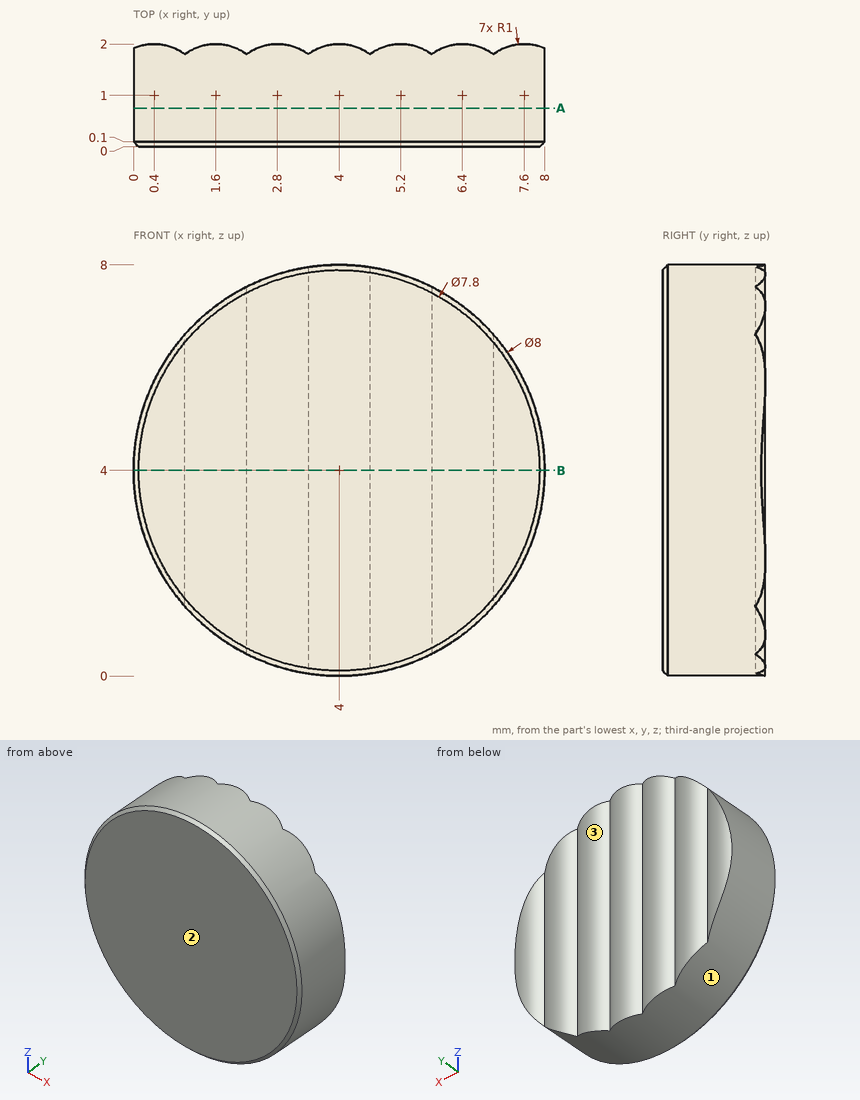
Design review of the part shown in the three views and the two pictorial views. Dimensions are in mm from the part's minimum x, y and z. Round coordinates to 2 decimals unless told otherwise and drop trailing zeros. Loops run counter-clockwise (first coordinate to the right, second up) from the corner with the lowest first, then second, coordinate; pieces in that order, holes last. Notation, with made-up numbers: M -35,-14 L 11,-14 A17 cw 11,10 Z; hole C -32.5,-22 d5. An arc over 180 degrees is marked long. Put each result on its own line as item: value.
Q1. To check wall thickness, follow L1, parallel to Z at x = 7, y = 0.2; L2, parallel to Y at x = 0.75, z = 6; L3, parallel to Z at x = 3.5, y = 1.75. State the ranges of each line that lie inside material, in increasing order.
Result set:
L1: z = 1.35 to 6.65
L2: y = 0 to 1.94
L3: z = 0.03 to 7.97
Q2. Consider section A-A, the plane y = 0.75. Give the boundary of the cut face in (x, z), then the cut area to 3 significant figures.
Result set:
outline: C 4,4 d8
area: 50.3 mm²
Q3. Mouldability with a two-part tool opening along X and no side actions: class the marked faces 1, 2 and 3 as released by +X, released by -X, zero draft, split by the parting line, or undercut.
Result set:
face 1: split by the parting line
face 2: zero draft
face 3: undercut
Q4. Consider section B-B, the plane z = 4. Give the boundary of the cut face in (x, y), then the cut area to 3 significant figures.
Result set:
outline: M 0,0.1 L 0.1,0 L 7.9,0 L 8,0.1 L 8,1.92 A1 ccw 7,1.8 A1 ccw 5.8,1.8 A1 ccw 4.6,1.8 A1 ccw 3.4,1.8 A1 ccw 2.2,1.8 A1 ccw 1,1.8 A1 ccw 0,1.92 Z
area: 15.5 mm²
